Input: part model. Units: mm. Frame: model coordinates. A direction names the side the tool comes from. Give positions to 0.01 mm unless a question says otherwise; leave off trailing zeros. Loops run counter-clockwise (first coordinate to the right, second up) from the corner with the lowest first, then second, coordinate; pieces in that order, holes last. Notation, with made-up numbers: (-17.75, -7.75) - (6.25, -7.75) arc R16 ccw to (6.25, 4.25) - close; hole circle Ø3 at (80.5, 41.5). An arc over 180 degrees is marked (long way). Answer as a JSON object with one key per item and string values. Group by question number.
(1) Mould query, pull axis Y, two halves, no side actions, for faces 1 (the flat face through (-147, 10, 25.4)), 2 (the cylindrical face through (9.523, 9.316, 6.261)), 3 (the cylindrical face through (-98.91, 7.09, 6.44)). Classes: +Y half, -Y half, draft (parallel to the pull), parting line (faces both ways), or undercut.
(2) Section query B-B (z = 6). Return loops of the section in (x, y) (3 decimals), plus the area to 3 significant figures.
(3) Pin query (flat end, axial travel): P1, Ø3, axis at y = 7, z = 11.5, coming from the -X side; P2, Ø8, axis at x = -33, y = 10.5, coming from the +Z side; P3, Ø6, axis at x = -138, y = 8.5, coming from the -Z side. Return the tip coordinate at first contact, or that it passes through.
(4) Access query for faces 4 (the cylindrical face through (-141.158, 11.432, 18.961)), 5 (the cylindrical face through (-161.923, 9.734, 6.261)). Directions: +Z, -Z, +X, -X, +Y, -Y. A direction counts if a zero-diameter tool reaches every point of the face in a straight line with its end or side. Return the directions, or none.
(5) Material intervals for L1, parallel to Z at x = -106, y = 1.5; L2, parallel to X at y = 12.5, z = 8; L3, parallel to X at y = 12.75, z = 13.5, sorted ascending.
(6) Section query C-C (x = -54.5). Return loops of the section in (y, z), plus the area to 3 significant figures.
(7) Section query D-D (z = 20). Return loops of the section in (x, y) (3 decimals), plus the area to 3 significant figures.
(8) Section query A-A (y = 12.75). Return loops of the section in (x, z), plus the area to 3 significant figures.
```python
from build123d import *

# Parameters (mm, degrees)
F1_DEPTH = 12.7
F2_R     = 6.35
F3_DEPTH = 25.4
F4_R     = 6.35
F5_DEPTH = 12.7


with BuildPart() as f1:
    # F0 (on Top) → F1 (new body)
    with BuildSketch(Plane.XY):
        with BuildLine():
            Line((-152.4, 0), (0, 0))
            ThreePointArc((0, 0), (9.525, 9.525), (0, 19.05))
            Line((0, 19.05), (-152.4, 19.05))
            ThreePointArc((-152.4, 19.05), (-161.925, 9.525), (-152.4, 0))
        make_face()
    extrude(amount=F1_DEPTH)

    # F2 (on face) → F3 (cut)
    with BuildSketch(Plane.XY.offset(12.7)):
        with Locations((-104.775, 9.525)):
            Circle(F2_R)
        with Locations((-3.175, 9.525)):
            Circle(F2_R)
    extrude(amount=-F3_DEPTH, mode=Mode.SUBTRACT)

    # F4 (on face) → F5 (join)
    with BuildSketch(Plane.XY.offset(12.7)):
        with Locations((-147.214279, 9.525)):
            Circle(F4_R)
    extrude(amount=F5_DEPTH)


solid = f1.part
```
Recorded:
{
 "1": {"face 1": "draft", "face 2": "parting line", "face 3": "undercut"},
 "2": {"outline": "(-152.4, 0) - (0, 0) arc R9.525 ccw to (0, 19.05) - (-152.4, 19.05) arc R9.525 ccw to start; hole circle Ø12.7 at (-104.775, 9.525); hole circle Ø12.7 at (-3.175, 9.525)", "area": "2,930 mm^2"},
 "3": {"P1": "stops at x = -161.87", "P2": "stops at z = 12.7", "P3": "stops at z = 0"},
 "4": {"face 4": "+Z", "face 5": "+Z, -Z, -X"},
 "5": {"L1": "z = 0 to 12.7", "L2": "x = -161.45 to -110.38, -99.17 to -8.78, 2.43 to 9.05", "L3": "x = -152.68 to -141.74"},
 "6": {"outline": "(0, 0) - (19.05, 0) - (19.05, 12.7) - (0, 12.7) - close", "area": "242 mm^2"},
 "7": {"outline": "circle Ø12.7 at (-147.214, 9.525)", "area": "127 mm^2"},
 "8": {"outline": "(-161.36, 0) - (-110.25, 0) - (-110.25, 12.7) - (-141.74, 12.7) - (-141.74, 25.4) - (-152.68, 25.4) - (-152.68, 12.7) - (-161.36, 12.7) - close; (-99.3, 0) - (-8.65, 0) - (-8.65, 12.7) - (-99.3, 12.7) - close; (2.3, 0) - (8.96, 0) - (8.96, 12.7) - (2.3, 12.7) - close", "area": "2,020 mm^2"}
}
